Part model, mm, in its own coordinate system. A direction names the side the tool comes from. Give positions to 0.01 mm unless a question says otherwise; leave off trailing zeros. Order: outer loops, then holes, each group sorted by start corner. A loop starts at its lowest first (then second) coordinate and runs counter-clockwise, first axis right, second up. Notation, with made-up numbers: M 89,-38 L 103,-38 A20 ccw 103,-2 Z; hole C -15.5,32 d1. An arc over 180 degrees is marked long. Answer as a JSON object with one key per item and string values.
Autodesk Inventor part; units mm, degrees
ref_plane "YZ Plane" through (0, 0, 0) normal (1, 0, 0) x (0, 1, 0)
ref_plane "XZ Plane" through (0, 0, 0) normal (0, 1, 0) x (-1, 0, 0)
ref_plane "XY Plane" through (0, 0, 0) normal (0, 0, 1) x (1, 0, 0)
sketch "Sketch1" plane through (0, 0, 0) normal (0, 1, 0) x (-1, 0, 0)
  line L0 (0, 0) -> (60, 0)
  line L1 (60, 0) -> (60, -81)
  line L2 (60, -81) -> (0, -81)
  line L3 (0, -81) -> (0, 0)
  line L4 (45, -21.6284) -> (15, -21.6284) construction
  line L5 (45, -81) -> (45, 0) construction
  line L6 (15, 0) -> (15, -81) construction
  circle A0 centre (40, -73.5) radius 1.5
  circle A1 centre (40, -7.5) radius 1.5
  circle A2 centre (20, -7.5) radius 1.5
  circle A3 centre (20, -73.5) radius 1.5
  line L7 (60, -40.5) -> (0, -40.5) construction
  line L8 (30, 0) -> (30, -81) construction
  circle A4 centre (30, -40.5) radius 24
  circle A5 centre (30, -40.5) radius 27.5
  circle A6 centre (57.1293, -36) radius 1.5
  circle A7 centre (57.1293, -45) radius 1.5
  circle A8 centre (25.5, -13.3707) radius 1.5
  circle A9 centre (34.5, -13.3707) radius 1.5
  circle A10 centre (2.8707, -45) radius 1.5
  circle A11 centre (2.8707, -36) radius 1.5
  circle A12 centre (34.5, -67.6293) radius 1.5
  circle A13 centre (25.5, -67.6293) radius 1.5
  circle A14 centre (30, -40.5) radius 40 construction
  arc A15 (60, -81) -> (60, 0) centre (-17.0125, -40.5) ccw
  circle A16 centre (30, -40.5) radius 36.28 construction
  circle A17 centre (65.9998, -36) radius 1.5
  circle A18 centre (65.9998, -45) radius 1.5
  circle A19 centre (-5.9998, -45) radius 1.5
  circle A20 centre (-5.9998, -36) radius 1.5
  arc A21 (0, 0) -> (0, -81) centre (77.0125, -40.5) ccw
  line L9 (30, -40.5) -> (-3.3536, -73.8536) construction
  circle A22 centre (1.7157, -68.7843) radius 1.5
  circle A23 centre (11.8404, -76.1403) radius 1.5
  circle A24 centre (23.7426, -80.0075) radius 1.5
  circle A25 centre (36.2574, -80.0075) radius 1.5
  circle A26 centre (48.1596, -76.1403) radius 1.5
  circle A27 centre (58.2843, -68.7843) radius 1.5
  circle A28 centre (65.6403, -58.6596) radius 1.5
  circle A29 centre (69.5075, -46.7574) radius 1.5
  circle A30 centre (69.5075, -34.2426) radius 1.5
  circle A31 centre (65.6403, -22.3404) radius 1.5
  circle A32 centre (58.2843, -12.2157) radius 1.5
  circle A33 centre (48.1596, -4.8597) radius 1.5
  circle A34 centre (36.2574, -0.9925) radius 1.5
  circle A35 centre (23.7426, -0.9925) radius 1.5
  circle A36 centre (11.8404, -4.8597) radius 1.5
  circle A37 centre (1.7157, -12.2157) radius 1.5
  circle A38 centre (-5.6403, -22.3404) radius 1.5
  circle A39 centre (-9.5075, -34.2426) radius 1.5
  circle A40 centre (-9.5075, -46.7574) radius 1.5
  circle A41 centre (-5.6403, -58.6596) radius 1.5
  circle A42 centre (48.1596, -68.7843) radius 1.5
  circle A43 centre (48.1596, -12.2157) radius 1.5
  circle A44 centre (11.8404, -12.2157) radius 1.5
  circle A45 centre (11.8404, -68.7843) radius 1.5
  line L10 (0, 0) -> (6, 0)
  arc A46 (6, 0) -> (6.3936, -12.9505) centre (40.8143, -5.423) ccw
  arc A47 (6.3936, -12.9505) -> (-5.0141, -31) centre (30, -40.5) ccw
  line L11 (-9.4798, -31) -> (7.9603, -31)
  line L12 (-10, -40.5) -> (70, -40.5) construction
  line L13 (-18.775, -14.5) -> (-31.775, -14.5)
  line L14 (-31.775, -14.5) -> (-31.775, -24.5)
  line L15 (-31.775, -24.5) -> (-18.775, -24.5)
  line L16 (-18.775, -24.5) -> (-18.775, -14.5)
  line L17 (-18.775, -54.5) -> (-37.775, -54.5)
  line L18 (-37.775, -54.5) -> (-37.775, -68.5)
  line L19 (-37.775, -68.5) -> (-18.775, -68.5)
  line L20 (-18.775, -68.5) -> (-18.775, -54.5)
  line L21 (-17.0125, -40.5) -> (-69.0232, -40.5)
  line L22 (-16.775, -12.5) -> (-23.775, -12.5)
  line L23 (-23.775, -12.5) -> (-23.775, -26.5)
  line L24 (-23.775, -26.5) -> (-16.775, -26.5)
  line L25 (-16.775, -26.5) -> (-16.775, -12.5)
  line L26 (-16.775, -52.5) -> (-23.775, -52.5)
  line L27 (-23.775, -52.5) -> (-23.775, -70.5)
  line L28 (-23.775, -70.5) -> (-16.775, -70.5)
  line L29 (-16.775, -70.5) -> (-16.775, -52.5)
  circle A48 centre (-30.175, -16.1) radius 1.25
  circle A49 centre (-30.175, -22.9) radius 1.25
  circle A50 centre (-35.775, -56.5) radius 1.25
  line L30 (-16.775, -32.5) -> (-49.775, -32.5)
  line L31 (-51.775, -34.5) -> (-51.775, -46.5)
  line L32 (-49.775, -48.5) -> (-16.775, -48.5)
  line L33 (-16.775, -48.5) -> (-16.775, -32.5)
  line L34 (-16.775, -43.5) -> (-38.775, -43.5) construction
  line L35 (-32.0174, -32.5) -> (-46.0174, -32.5)
  line L36 (-46.0174, -32.5) -> (-46.0174, -48.5)
  line L37 (-46.0174, -48.5) -> (-32.0174, -48.5)
  line L38 (-32.0174, -48.5) -> (-32.0174, -32.5)
  line L39 (0, 0) -> (-59.1614, -10.4318)
  line L40 (0, -81) -> (-59.1614, -70.5682)
  arc A51 (-51.775, -9.1293) -> (-51.775, -71.8707) centre (29.3856, -40.5) ccw
  arc A52 (-49.775, -32.5) -> (-51.775, -34.5) centre (-49.775, -34.5) ccw
  arc A53 (-51.775, -46.5) -> (-49.775, -48.5) centre (-49.775, -46.5) ccw
  arc A54 (6.3936, -68.0495) -> (6, -81) centre (40.8143, -75.577) ccw
  arc A55 (-5.0141, -50) -> (6.3936, -68.0495) centre (30, -40.5) ccw
  line L41 (-9.4798, -50) -> (7.9603, -50)
  arc A56 (-4.4033, -0.7764) -> (-4.4033, -80.2236) centre (73.0125, -40.5) ccw
  circle A57 centre (1.7157, -12.2157) radius 3.25
  circle A58 centre (1.7157, -68.7843) radius 3.25
  arc A59 (6.3936, -12.9505) -> (7.0417, -15.4657) centre (40.8143, -5.423) ccw
  arc A60 (7.0417, -15.4657) -> (0, -20.0981) centre (14.8139, -34.9486) ccw
  arc A61 (7.0417, -65.5343) -> (6.3936, -68.0495) centre (40.8143, -75.577) ccw
  arc A62 (0, -60.9019) -> (7.0417, -65.5343) centre (14.8139, -46.0514) ccw
  point P0 (30, -21.6284)
  point P1 (-18.775, -19.5)
  point P2 (-18.775, -61.5)
  point P3 (-51.775, -48.5)
  point P4 (-51.775, -32.5)
  point P5 (-16.775, -40.5)
  point P6 (-16.775, -61.5)
  point P7 (-51.775, -40.5)
  point P8 (-14, -40.5)
  point P9 (6, -81)
  point P10 (0, -60.9019)
  dimension "d18" = 48
  dimension "d6" = 60
  dimension "d7" = 81
  dimension "d8" = 3
  dimension "d9" = 7.5
  dimension "d10" = 5
  dimension "d11" = 30
  dimension "d12" = 3
  dimension "d13" = 7.5
  dimension "d14" = 5
  dimension "d15" = 3
  dimension "d16" = 3
  dimension "d17" = 5
  dimension "d19" = 55
  dimension "d20" = 3
  dimension "d21" = 4.5
  dimension "d22" = 3
  dimension "d23" = 4.5
  dimension "d24" = 360
  dimension "d25" = 80
  dimension "d26" = 72.56
  dimension "d27" = 3
  dimension "d28" = 3
  dimension "d29" = 360
  dimension "d30" = 45
  dimension "d31" = 3
  dimension "d32" = 360
  dimension "d33" = 3
  dimension "d34" = 3
  dimension "d35" = 3
  dimension "d36" = 3
  dimension "d37" = 6
  dimension "d38" = 5
  dimension "d39" = 30
  dimension "d40" = 40.5
  dimension "d41" = 13
  dimension "d42" = 10
  dimension "d43" = 19
  dimension "d44" = 14
  dimension "d45" = 7
  dimension "d46" = 2
  dimension "d47" = 2
  dimension "d48" = 2
  dimension "d49" = 2
  dimension "d50" = 2
  dimension "d51" = 2
  dimension "d52" = 7
  dimension "d53" = 2.5
  dimension "d54" = 2.5
  dimension "d55" = 1.6
  dimension "d56" = 1.6
  dimension "d57" = 2.5
  dimension "d58" = 2
  dimension "d59" = 2
  dimension "d60" = 35
  dimension "d61" = 16
  dimension "d62" = 4
  dimension "d63" = 6
  dimension "d64" = 22
  dimension "d65" = 14
  dimension "d66" = 80
  dimension "d67" = 80
  dimension "d68" = 2
  dimension "d69" = 4
  dimension "d78" = 6.5
extrude "Extrusion1" add sketch "Sketch1" along normal blind 2 contours L0 A46 A47 L3 A57 | L3 A57 A47 L11 A21 | A21 A39 A40 L40 A56 L39 | A59 A60 A47 | A21 A39 | L3 A58 A55 A54 L2 | A21 L41 A55 L3 A58 | A21 A40 | A62 A61 A55 picked at (-10.1825, -34.1938) picked at (-10.1825, -46.8062)
extrude "Extrusion2" add sketch "Sketch1" against normal blind 4 contours A21 A39 A40 L40 A56 L39 | A21 A39 | A21 A40 picked at (-10.1825, -34.1938) picked at (-10.1825, -46.8062)
ref_plane "Work Plane1" through (0, -5.5, 0) normal (0, -1, 0) x (1, 0, 0)
sketch "Sketch2" plane through (0, -5.5, 0) normal (0, -1, 0) x (1, 0, 0)
  line L0 (0, -81) -> (59.1614, -70.5682)
  arc A0 (51.775, -71.8707) -> (51.775, -9.1293) centre (-29.3856, -40.5) ccw
  line L1 (49.775, -48.5) -> (16.775, -48.5)
  arc A1 (49.775, -48.5) -> (51.775, -46.5) centre (49.775, -46.5) ccw
  line L2 (51.775, -34.5) -> (51.775, -46.5)
  arc A2 (51.775, -34.5) -> (49.775, -32.5) centre (49.775, -34.5) ccw
  line L3 (16.775, -32.5) -> (49.775, -32.5)
  line L4 (46.0174, -32.5) -> (46.0174, -48.5)
  line L5 (32.0174, -48.5) -> (32.0174, -32.5)
  line L6 (16.775, -48.5) -> (16.775, -32.5)
  arc A3 (4.4033, -80.2236) -> (4.4033, -0.7764) centre (-73.0125, -40.5) ccw
  arc A4 (0, -81) -> (0, 0) centre (-77.0125, -40.5) ccw
  line L7 (37.775, -68.5) -> (18.775, -68.5)
  line L8 (37.775, -54.5) -> (37.775, -68.5)
  line L9 (18.775, -54.5) -> (37.775, -54.5)
  circle A5 centre (35.775, -56.5) radius 1.25
  line L10 (23.775, -52.5) -> (23.775, -70.5)
  line L11 (23.775, -70.5) -> (16.775, -70.5)
  line L12 (16.775, -70.5) -> (16.775, -52.5)
  line L13 (18.775, -68.5) -> (18.775, -54.5)
  line L14 (16.775, -52.5) -> (23.775, -52.5)
  line L15 (31.775, -24.5) -> (18.775, -24.5)
  line L16 (31.775, -14.5) -> (31.775, -24.5)
  circle A6 centre (30.175, -16.1) radius 1.25
  line L17 (18.775, -14.5) -> (31.775, -14.5)
  line L18 (0, 0) -> (59.1614, -10.4318)
  line L19 (23.775, -12.5) -> (23.775, -26.5)
  line L20 (16.775, -12.5) -> (23.775, -12.5)
  line L21 (16.775, -26.5) -> (16.775, -12.5)
  line L22 (18.775, -24.5) -> (18.775, -14.5)
  line L23 (23.775, -26.5) -> (16.775, -26.5)
  line L24 (17.0125, -40.5) -> (69.0232, -40.5)
  point P0 (23.775, -24.5)
  point P1 (23.775, -14.5)
  point P2 (23.775, -68.5)
  point P3 (23.775, -54.5)
extrude "Extrusion3" add sketch "Sketch2" along normal blind 2.5 contours A4 L18 A3 L0 | L2 A1 L1 L4 L24 | L24 L4 L3 A2 L2 | A3 L18 A0 L0 | L5 L1 L6 L3 | L7 L10 L9 L8 | L15 L19 L17 L16
extrude "Extrusion4" add sketch "Sketch2" against normal up to surface (1.5 mm away) contours A4 L18 A3 L0
fillet "Fillet1" radius 2 3 edges at (46.0174, -6.75, -32.5) (46.0174, -6.75, -48.5) (14, -5.5, -40.5)
fillet "Fillet2" radius 15 2 edges at (0, 1, -20.0981) (0, 1, -60.9019)
sketch "Sketch3" plane through (0, 2, 0) normal (0, 1, 0) x (1, 0, 0)
  arc A0 (-6, 0) -> (-7.0417, 15.4657) centre (-40.8143, 5.423) ccw
  line L0 (-5.5916, 6.3226) -> (7.0067, 6.3226)
  arc A1 (4.4033, 0.7764) -> (4.4033, 80.2236) centre (-73.0125, 40.5) ccw
  line L1 (7.0067, 6.3226) -> (36.6975, 11.5578)
  arc A2 (51.775, 9.1293) -> (51.775, 71.8707) centre (-29.3856, 40.5) ccw
  line L2 (51.775, 9.1293) -> (6.8591, 1.2095)
  line L3 (36.6975, 11.5578) -> (36.6975, 31)
  line L4 (9.4798, 31) -> (5.0141, 31)
  line L5 (5.0141, 31) -> (36.6975, 31)
  arc A3 (1.5276, 22.5487) -> (5.0141, 31) centre (-30, 40.5) ccw
  arc A4 (-3.2083, 17.4758) -> (1.5276, 22.5487) centre (-11.5075, 29.9707) ccw
  arc A5 (-7.0417, 15.4657) -> (-3.2083, 17.4758) centre (-14.8139, 34.9486) ccw
  line L6 (-14.8139, 83.8993) -> (60.693, 83.8993)
  line L7 (60.693, 83.8993) -> (60.693, -4.0621)
  line L8 (60.693, -4.0621) -> (-14.8139, -4.0621)
  line L9 (-14.8139, -4.0621) -> (-14.8139, 83.8993)
  point P0 (0, 0)
extrude "Extrusion5" cut sketch "Sketch3" against normal up to surface (10 mm away)
equation "\"d11\" = 0.5 * d6"
equation "\"d12\" = d8"
equation "\"d15\" = d8"
equation "\"d16\" = d8"
equation "\"d22\" = d8"
equation "\"d27\" = d8"
equation "\"d28\" = d8"
equation "\"d31\" = d8"
equation "\"d33\" = d8"
equation "\"d34\" = d8"
equation "\"d35\" = d8"
equation "\"d36\" = d8"
properties part number "SensorHolderSmall"
1. Which spindle directions (+Z, -Z, +X, -X, +Y, -Y) get a long thin tool onto all of the face, cutting with end or side? Do faces 4 (the flat face through (3, 2, -18)), 5 (the flat face through (3, 0, -18)), 6 (the flat face through (26, -5.5, -19)), 7 (the flat face through (23.775, -7, -19)). Say none if no direction does.
Worked answers:
{"face 4": "+Z, -Z, +X, -X, +Y", "face 5": "-Z, -X, -Y", "face 6": "+Z, +X, +Y", "face 7": "+Y, -Y"}
2. Cut at B-B on x = 31. Give the cut face in (y, z).
Worked answers:
{"outline": "M -8,-31 L -5.5,-31 L -5.5,-17.04 L -8,-17.04 Z; M -8,-15.16 L -5.5,-15.16 L -5.5,-10.55 L -8,-10.55 Z"}
3. Cut at A-A on y = -7. State how many separate pieces and enclosed holes the cut face has, plus the area to 3 significant figures.
Worked answers:
{"separate pieces": "1", "enclosed holes": "2", "area": "555 mm^2"}
4. Cut at D-D on y = -3. Give the cut face in (x, z) (1 decimal), plus the area to 3 significant figures.
Worked answers:
{"outline": "M 3,-6.3 A87 cw 9.5,-31 L 13.5,-31 A87 ccw 7,-6.3 Z", "area": "98.7 mm^2"}
5. Two-plate mould, pull along Z, no slides. Class faces 1 (the cylindrical face through (-6.7, 0.99, -14.23)), 2 (the cylindrical face through (3.51, 1.01, -26.6)), 3 (the cylindrical face through (-1.293, 0.986, -15.438)): +Z half, -Z half, draft (parallel to the pull), parting line (faces both ways), or undercut.
Worked answers:
{"face 1": "+Z half", "face 2": "-Z half", "face 3": "undercut"}
6. Pin check, flat tips, straight feed: P1, Ø1.2, axis at x = 21, y = -7, coming from the +Z side; P2, Ø4, axis at x = 30.175, z = -16.1, coming from the -Y side; P3, Ø7.5, axis at x = 22, z = -22.5, coming from the +Y side; P4, Ø8.5, axis at x = -1.72, z = -12.22, coming from the -Y side. Stop position of each tip, or through.
Worked answers:
{"P1": "stops at z = -8.68", "P2": "stops at y = -8", "P3": "stops at y = -5.5", "P4": "stops at y = 0"}
7. Probe line 1 along Y through (x, z) = (13, -14.5); line 2 along X through (y, z) = (1, -12); line 3 along Y through (x, z) = (3, -7.5). List the from-to ranges inside material, lowest first.
Worked answers:
{"line 1": "y = -8 to -5.5", "line 2": "x = -6.2 to -4.96, 1.53 to 9.2", "line 3": "y = 0 to 2"}
